Geometry: final body of the model. Coordinates: model frame, mm. A direction names the side the tool comes from. Round coordinates to 2 decimals unless told otherwise and drop trailing zeros. Loops run counter-clockwise (first coordinate to the right, second up) from the corner with the lowest first, then second, coordinate; pieces in that order, holes last. Notation, with made-up numbers: (1, -23.75) - (28, -23.75) arc R23 cw to (28, 0.25) - close; hole circle Ø5 at (49, -11). An arc over 180 degrees is marked (long way). Answer in a Markdown table with one row per item. Add a question column.
from build123d import *

# Parameters (mm, degrees)
F0_W     = 1.5
F0_H     = 56
F3_DEPTH = 25


with BuildPart() as f1:
    # F0 (on Front) → F1 (revolve)
    with BuildSketch(Plane.XZ):
        with BuildLine():
            ThreePointArc((-12.5, 56), (-8.8388347648, 64.8388347648), (0, 68.5))
            Line((0, 68.5), (0, 70))
            ThreePointArc((0, 70), (-9.8994949366, 65.8994949366), (-14, 56))
            Line((-14, 56), (-12.5, 56))
        make_face()
        with Locations((-13.25, 28)):
            Rectangle(F0_W, F0_H)
    revolve(axis=Axis((0, 0, 28), (0, 0, -1)))

    # F2 (on Front) → F3 (cut)
    with BuildSketch(Plane.XZ):
        with BuildLine():
            Line((6, -2.9855446036), (6, 48))
            ThreePointArc((6, 48), (0, 54), (-6, 48))
            Line((-6, 48), (-6, -2.9855446036))
            Line((-6, -2.9855446036), (6, -2.9855446036))
        make_face()
    extrude(amount=F3_DEPTH, mode=Mode.SUBTRACT)


solid = f1.part
1) Section D-D, the plane z = 13.5. Return the cut outline in (x, y), and give its area (3 significant figures).
2) Pull-direction query (X, two-part tool) for faces 1 (the flat face through (0, 13, 0)), 2 (the flat face through (-6, -12, 24)), 3 (the cylindrical face through (0, -13, 54)), 4 (the cylindrical face through (-7.526, 11.805, 28.392)); classes: pulls with the +X half, pulls with the -X half, needs draft (parallel to the pull), parting line crosses it, or undercut.
3) Section A-A, the plane y = 0. Return the cut outline in (x, z), and give its area (3 significant figures).
4) Contact query for flat-ended pins moving along their axis: pin 1 Ø0.5 at (y, z) = (-12, 14) entering from -X; pin 2 Ø5 at (y, z) = (-8, 31) entering from +X; pin 3 Ø8 at (y, z) = (-10.5, 41.5) entering from -X. Output: stop coordinate, or through.
5) Section B-B, the plane x = 0. Return the cut outline in (y, z), and give its area (3 significant figures).
6) Material intervals for line 1 along X through (y, z) = (0, 21); line 2 along Y through (x, z) = (0, 29.5); line 3 along X through (y, z) = (9, 38), sorted ascending. Write a range as from..to.
7) Section C-C, the plane z = 60. Return the cut outline in (x, y).
8) Reachability of faces 5 (the flat face through (6, -12, 24)), 6 (the cylindrical face through (1.627, 12.394, 28.392)) from +Z, -Z, +X, -X, +Y, -Y: full face, straight path, thin tool, end or side. Return the list, or none.
Evaluation:
| question | item | result |
|---|---|---|
| 1 | outline | (-6, -12.65) - (-6, -10.97) arc R12.5 cw (long way) to (6, -10.97) - (6, -12.65) arc R14 ccw (long way) to start |
| 1 | area | 106 mm² |
| 2 | face 1 | needs draft |
| 2 | face 2 | undercut |
| 2 | face 3 | undercut |
| 2 | face 4 | parting line crosses it |
| 3 | outline | (-14, 0) - (-12.5, 0) - (-12.5, 56) arc R12.5 cw to (12.5, 56) - (12.5, 0) - (14, 0) - (14, 56) arc R14 ccw to (-14, 56) - close |
| 3 | area | 230 mm² |
| 4 | pin 1 | stops at x = -7.61 |
| 4 | pin 2 | stops at x = 12.87 |
| 4 | pin 3 | stops at x = -12.4 |
| 5 | outline | (-14, 54) - (-12.5, 54) - (-12.5, 56) arc R12.5 cw to (12.5, 56) - (12.5, 0) - (14, 0) - (14, 56) arc R14 ccw to (-14, 56) - close |
| 5 | area | 149 mm² |
| 6 | line 1 | x = -14..-12.5, 12.5..14 |
| 6 | line 2 | y = 12.5..14 |
| 6 | line 3 | x = -10.72..-8.67, 8.67..10.72 |
| 7 | outline | circle Ø26.83 at (0, 0); hole circle Ø23.69 at (0, 0) |
| 8 | face 5 | -Z, -Y |
| 8 | face 6 | -Z |
